Geometry check sheet. Reference: the model listing, model coordinates, mm. Face numbers are marked on the shaded views. Round coordinates to 2 decimals unless told otherwise and drop trailing zeros. Write each loop counter-clockwise with the first axis right and the second up, starting at its lowest first coordinate (ties: lowest second). Pieces come first, ordered by that corner, then holes. Notation, with made-up numbers: M 50.5,36.5 L 70.5,36.5 A21 ccw 70.5,42.5 Z; hole C 37.25,57.5 d1. An arc over 180 degrees is marked long. One line per item, written item: value. Start each with the question number.
1. Section check C-C (x = 13). Record the boundary of the cut face in (y, z).
2. Release check for a two-part mould opening along Z. For the marked faces 1 and 2 record: pulls with the +Z half, pulls with the -Z half, needs draft (parallel to the pull), parting line crosses it, or undercut.
3. Section check A-A (y = 4.25). Record the boundary of the cut face in (x, z), and give its area (3 significant figures).
4. Scan lines: probe 1 along Z at (x, y) = (21.45, 4.25); probe 2 along X at (y, z) = (4, 39.9); probe 3 along Z at (x, y) = (-21.45, 4.75). Record each from-to range of solid material in increasing order. Write a range as [from, to].
5. Section check D-D (z = 6.5). Record the boundary of the cut face in (x, y), and give its area (3 significant figures).
6. Depth check by flat-ended pin: P1, Ø4, axis at x = 17, z = -11, coming from the +Y side; P2, Ø1.8, axis at x = 8.5, y = 4, coming from the +Z side; P3, Ø3, axis at y = 3.5, z = 14.5, coming from the -X side; P4, Ø2.5, axis at x = -21.45, z = 39.9, coming from the +Y side. Enter the tip coordinate at first touch or a pass-through.
7. Section check B-B (z = -23). Record the boundary of the cut face in (x, y).
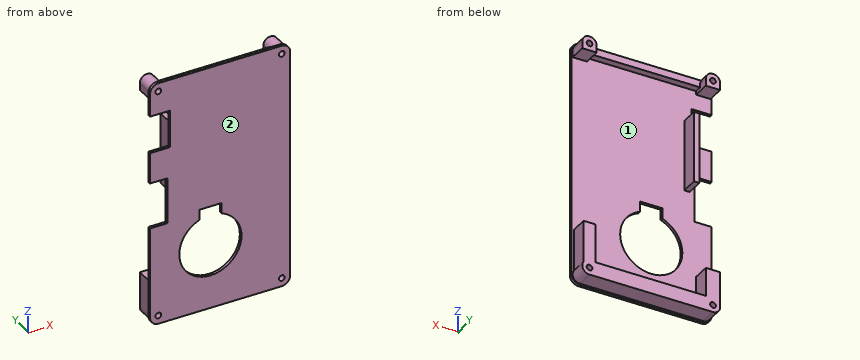
Autodesk Inventor part; units mm, degrees
ref_plane "YZ Plane" through (0, 0, 0) normal (1, 0, 0) x (0, 1, 0)
ref_plane "XZ Plane" through (0, 0, 0) normal (0, 1, 0) x (-1, 0, 0)
ref_plane "XY Plane" through (0, 0, 0) normal (0, 0, 1) x (1, 0, 0)
sketch "Sketch1" plane through (0, 0, 0) normal (0, 1, 0) x (-1, 0, 0)
  line L0 (-21.35, 42.8) -> (21.35, 42.8)
  line L1 (24.35, 39.8) -> (24.35, -39.8)
  line L2 (21.35, -42.8) -> (-21.35, -42.8)
  line L3 (-24.35, -39.8) -> (-24.35, 39.8)
  arc A0 (24.35, 39.8) -> (21.35, 42.8) centre (21.35, 39.8) ccw
  arc A1 (21.35, -42.8) -> (24.35, -39.8) centre (21.35, -39.8) ccw
  arc A2 (-24.35, -39.8) -> (-21.35, -42.8) centre (-21.35, -39.8) ccw
  arc A3 (-21.35, 42.8) -> (-24.35, 39.8) centre (-21.35, 39.8) ccw
  line L4 (-47.6975, 0) -> (69.2667, 0) construction
  point P0 (0, 0)
  dimension "d2" = 3
sketch "Sketch2" plane through (0, 0, 0) normal (0, 1, 0) x (-1, 0, 0)
  line L0 (-24.35, 42.8) -> (24.35, -42.8) construction
  line L1 (24.35, 42.8) -> (-24.35, -42.8) construction
  circle A0 centre (21.45, 39.9) radius 1
  line L2 (0, 76.772) -> (0, -116.4578) construction
  circle A1 centre (21.45, 39.9) radius 2.5
  line L3 (19.2849, 41.15) -> (-19.2849, 41.15)
  line L4 (-19.2849, 41.15) -> (-19.2849, 38.65)
  line L5 (-19.2849, 38.65) -> (19.2849, 38.65)
  line L6 (19.2849, 38.65) -> (19.2849, 41.15)
  circle A2 centre (-21.45, 39.9) radius 2.5
  circle A3 centre (-21.45, 39.9) radius 1
  line L7 (23.95, 39.9) -> (18.95, 39.9)
  line L8 (18.95, 39.9) -> (18.95, 37.4)
  line L9 (18.95, 37.4) -> (23.95, 37.4)
  line L10 (-23.95, 39.9) -> (-18.95, 39.9)
  line L11 (-18.95, 37.4) -> (-23.95, 37.4)
  line L12 (-18.95, 39.9) -> (-18.95, 37.4)
  line L13 (24.35, 39.8) -> (24.35, -39.8)
  line L14 (-21.35, 42.8) -> (21.35, 42.8)
  arc A4 (24.35, 39.8) -> (21.35, 42.8) centre (21.35, 39.8) ccw
  line L15 (23.95, 39.9) -> (23.95, 37.4)
  line L16 (-23.95, 37.4) -> (-23.95, 39.9)
  point P0 (0, 0)
  point P1 (0, 0)
  point P2 (-21.35, 39.8)
  point P3 (21.45, 39.9)
  point P4 (-18.95, 38.65)
  point P5 (18.95, 38.65)
  point P6 (-21.45, 37.4)
  dimension "d16" = 48.7
  dimension "d17" = 2
  dimension "d18" = 5
  dimension "d19" = 2.5
  dimension "d20" = 2.5
  dimension "d23" = 2.9
  dimension "d24" = 2.9
  dimension "d25" = 2.9
sketch "Sketch4" plane through (0, 0, 0) normal (0, 1, 0) x (-1, 0, 0)
  circle A0 centre (21.45, -39.9) radius 2.5
  circle A1 centre (21.45, -39.9) radius 1
  circle A2 centre (-21.45, -39.9) radius 1
  circle A3 centre (-21.45, -39.9) radius 2.5
  line L0 (23.95, -39.9) -> (18.95, -39.9)
  line L1 (18.95, -39.9) -> (18.95, -27.4467)
  line L2 (18.95, -27.4467) -> (23.95, -27.4467)
  line L3 (23.95, -27.4467) -> (23.95, -39.9)
  line L4 (21.45, -37.4) -> (-21.45, -37.4)
  line L5 (-21.45, -37.4) -> (-21.45, -42.4)
  line L6 (-21.45, -42.4) -> (21.45, -42.4)
  line L7 (21.45, -42.4) -> (21.45, -37.4)
  line L8 (-19.377, -38.5026) -> (-23.523, -38.5026)
  line L9 (-23.523, -38.5026) -> (-23.523, -23.9)
  line L10 (-23.523, -23.9) -> (-19.377, -23.9)
  line L11 (-19.377, -23.9) -> (-19.377, -38.5026)
  point P0 (0, 0)
  point P1 (21.35, -42.8)
  point P2 (24.35, -39.8)
  point P3 (21.35, -39.8)
  point P4 (-24.35, -39.8)
  point P5 (-21.35, -42.8)
  point P6 (-21.35, -39.8)
  point P7 (18.95, -37.4)
  point P8 (-19.377, -37.4)
  point P9 (-21.45, -23.9)
  point P10 (-21.45, -39.9)
  dimension "d52" = 16
sketch "Sketch5" plane through (0, 0, 0) normal (0, 1, 0) x (-1, 0, 0)
  line L0 (24.35, 39.8) -> (24.35, -39.8)
  line L1 (24.35, 8) -> (18.35, 8)
  line L2 (18.35, 8) -> (18.35, -8)
  line L3 (18.35, -8) -> (24.35, -8)
  line L4 (24.35, -8) -> (24.35, 8)
  line L5 (31.157, 0) -> (-16.4919, 0)
  point P0 (0, 0)
  point P1 (18.35, 0)
  point P2 (21.35, -8)
  dimension "d21" = 16
  dimension "d22" = 6
extrude "Extrusion2" add sketch "Sketch1" against normal blind 1
extrude "Extrusion3" add sketch "Sketch2" along normal blind 2.5 contours A1 L8 L5 L12 A2 L3
extrude "Extrusion4" add sketch "Sketch2" along normal blind 5.9 contours L7 A1 L6 A0 | A0 L7 L6 A1 | L15 L9 A1 | L7 A1 L6 | L6 A1 L7 | L9 L8 L5 A1 | L5 L8 A1 | A2 L10 L4 | L4 L10 A3 A2 | L10 A2 L4 | L4 A2 L10 A3 | L12 L5 A2 | A2 L11 L16 | L12 L11 A2 L5
extrude "Extrusion5" add sketch "Sketch4" along normal up to surface (5.9 mm away) contours L0 A1 L7 A0 | A0 L7 A1 L0 | A0 L4 L1 L2 L3 | L7 A1 L0 A0 | A0 L1 L4 | L6 A3 L11 L4 L1 A0 | A0 L0 A1 L7 | L5 A2 L8 A3 | A3 L8 L5 A2 | L11 A3 L4 | L4 A3 L9 L10 L11 | A3 L5 L8 | A3 L8 L5
extrude "Extrusion6" cut sketch "Sketch4" along normal through all both and the other way through all contours L0 L7 A1 | A1 L7 L0 | L7 L0 A1 | A1 L0 L7 | L5 A2 | A2 L5
extrude "Extrusion7" cut sketch "Sketch2" along normal through all both and the other way through all contours L7 A0 | A0 L7 | L10 A3 | A3 L10
extrude "Extrusion8" cut sketch "Sketch5" along normal through all both and the other way through all
sketch "Sketch6" plane through (0, -1, 0) normal (0, -1, 0) x (1, 0, 0)
  arc A0 (5.4227, -14.164) -> (0.5528, -10.3702) centre (-3.3726, -20.4316) ccw
  line L0 (0.5528, -10.3702) -> (0.5528, -6.679)
  line L1 (0.5528, -6.679) -> (-2.7471, -6.679)
  line L2 (-2.7471, -6.679) -> (-3.9471, -6.679)
  line L3 (-3.9471, -6.679) -> (-7.1971, -6.679)
  line L4 (-7.1971, -6.679) -> (-7.1971, -10.3315)
  arc A1 (-7.1971, -10.3315) -> (-12.1679, -14.164) centre (-3.3726, -20.4316) ccw
  arc A2 (-12.45, -14.5801) -> (-13.3806, -16.3723) centre (-3.3726, -20.4316) ccw
  arc A3 (-13.4465, -16.5387) -> (-13.4465, -24.3246) centre (-3.3726, -20.4316) ccw
  arc A4 (-13.3806, -24.491) -> (-12.45, -26.2832) centre (-3.3726, -20.4316) ccw
  arc A5 (-12.1679, -26.6992) -> (5.4227, -26.6992) centre (-3.3726, -20.4316) ccw
  arc A6 (5.7048, -26.2832) -> (6.6355, -24.491) centre (-3.3726, -20.4316) ccw
  arc A7 (6.7014, -24.3246) -> (6.7014, -16.5387) centre (-3.3726, -20.4316) ccw
  arc A8 (6.6355, -16.3723) -> (5.7048, -14.5801) centre (-3.3726, -20.4316) ccw
  arc A9 (-7.1971, -10.3315) -> (0.5528, -10.3702) centre (-3.3726, -20.4316) ccw
  point P0 (0, 0)
  point P1 (-13.3806, -24.491)
  point P2 (-12.45, -26.2832)
  point P3 (-12.1679, -26.6992)
  point P4 (5.7048, -26.2832)
  point P5 (6.6355, -24.491)
  point P6 (6.7014, -24.3246)
  point P7 (6.6355, -16.3723)
  point P8 (5.7048, -14.5801)
  point P9 (5.4227, -14.164)
extrude "Extrusion9" cut sketch "Sketch6" along normal through all both and the other way through all
sketch "Sketch7" plane through (0, -1, 0) normal (0, -1, 0) x (1, 0, 0)
  line L0 (-9.9467, 38.1508) -> (9.6849, 38.1508) construction
  line L1 (9.6849, 38.1508) -> (9.6849, 29.6438) construction
  line L2 (9.6849, 29.6438) -> (-9.9467, 29.6438) construction
  line L3 (-9.9467, 29.6438) -> (-9.9467, 38.1508) construction
  point P0 (0, 0)
sketch "Sketch8" plane through (0, -1, 0) normal (0, -1, 0) x (1, 0, 0)
  line L0 (-24.35, 39.8) -> (-24.35, -39.8)
  line L1 (-24.35, 8) -> (-24.35, 39.8)
  line L2 (-24.35, 18.8) -> (-17.35, 18.8)
  line L3 (-17.35, 18.8) -> (-17.35, 31.8)
  line L4 (-17.35, 31.8) -> (-24.35, 31.8)
  line L5 (-24.35, 31.8) -> (-24.35, 18.8)
  line L6 (21.35, 42.8) -> (-21.35, 42.8)
  point P0 (0, 0)
  dimension "d43" = 7
  dimension "d45" = 24
  dimension "d46" = 11
extrude "Extrusion10" cut sketch "Sketch8" along normal through all both and the other way through all
sketch "Sketch9" plane through (0, 0, 0) normal (0, 1, 0) x (1, 0, 0)
  line L0 (-14.8468, -26.7931) -> (-16.7148, -26.7931)
  line L1 (-16.7148, -26.7931) -> (-16.7148, -2.0705)
  line L2 (-16.7148, -2.0705) -> (-14.8468, -2.0705)
  line L3 (-14.8468, -2.0705) -> (-14.8468, -26.7931)
  point P0 (0, 0)
extrude "Extrusion11" add sketch "Sketch9" along normal up to surface (5.9 mm away)
properties part number "my_back_metric"
Result sheet:
1. outline: M -1,-42.8 L 0,-42.8 L 0,-42.4 L 5.9,-42.4 L 5.9,-37.4 L 0,-37.4 L 0,38.65 L 2.5,38.65 L 2.5,41.15 L 0,41.15 L 0,42.8 L -1,42.8 Z
2. face 1: undercut
2. face 2: needs draft
3. outline: M -23.95,-39.9 A2.5 ccw -21.45,-42.4 L 21.45,-42.4 A2.5 ccw 23.52,-38.5 L 23.52,-23.9 L 19.38,-23.9 L 19.38,-37.4 L -18.95,-37.4 L -18.95,-27.45 L -23.95,-27.45 Z; M -23.95,37.4 L -18.95,37.4 L -18.95,39.9 A2.5 ccw -23.95,39.9 Z; M -16.71,2.07 L -14.85,2.07 L -14.85,26.79 L -16.71,26.79 Z; M 18.95,37.4 L 23.95,37.4 L 23.95,39.9 A2.5 ccw 18.95,39.9 Z; hole C -21.45,-39.9 d2; hole C -21.45,39.9 d2; hole C 21.45,-39.9 d2; hole C 21.45,39.9 d2
3. area: 420 mm2
4. probe 1: z = [-42.4, -40.9], [-38.9, -23.9], [37.4, 38.9], [40.9, 42.4]
4. probe 2: x = [-23.95, -22.45], [-20.45, -18.95], [18.95, 20.45], [22.45, 23.95]
4. probe 3: z = [-42.4, -40.9], [-38.9, -27.45], [37.4, 38.9], [40.9, 42.4]
5. outline: M -18.35,-1 L 24.35,-1 L 24.35,0 L -14.85,0 L -14.85,5.9 L -16.71,5.9 L -16.71,0 L -18.35,0 Z
5. area: 53.7 mm2
6. P1: stops at y = 0
6. P2: stops at z = -37.4
6. P3: stops at x = -16.71
6. P4: stops at y = 5.9
7. outline: M -24.35,-1 L -13.86,-1 L -13.86,0 L -24.35,0 Z; M 7.12,-1 L 24.35,-1 L 24.35,0 L 7.12,0 Z
